Check sheet for the modelled part. Datum: model origin and axes. Units: mm. A direction names the side the tool comes from. Give positions to 0.01 mm unless a question says otherwise; leave off trailing zeros. Write each loop counter-clockwise with the first axis right and the second up, starting at its lowest first coordinate (ties: lowest second). Pieces come first, ordered by that corner, then holes. Notation, with made-up numbers: M 86.5,-11 L 121.5,-11 A25 ccw 121.5,19 Z; hole C 29,76.25 d2. An arc over 180 degrees is marked long. Write item = value, one per line. Start each with the question number.
1) Scan lines: line 1 along Z through (x, y) = (10, 39.5); line 2 along Z through (x, y) = (12, 28); line 3 along Y through (x, z) = (17, 18.75). Record each from-to range of solid material in increasing order. Write a range as [from, to].
2) Mould release check, pull along Y, two halves, no side actions. Record for faces 1 (the flat face through (1, 16.1, 1)), 2 (the flat face through (20, 39, 8)): released by +Y, released by -Y, zero draft, split by the parting line, or undercut.
3) Cross-section at D-D, the plane y = 33. Record the cut outline in (x, z).
4) Cross-section at A-A, the plane x = 10. Record the cut outline in (y, z), plus the area to 3 significant figures.
5) Access from +Z, -Z, +X, -X, +Y, -Y to the whole of each face (thin tool, end or side, straight path). Record for faces 3 (the cylindrical face through (16.88, 16.56, 0.76)), 4 (the cylindrical face through (3.12, 25.24, 0.76)), 5 (the flat face through (0, 39, 8)).
6) Cross-section at C-C, the plane x = 15.5. Record the cut outline in (y, z).
7) Cross-section at B-B, the plane z = 11.5. Record the cut outline in (x, y).
8) Go/stop test with flat-tipped pins: pin 1 (1.5 mm diameter, centred on x = 8, z = 3, fed in from -Y); pin 2 (6 mm diameter, centred on x = 14, y = 14.5, fed in from +Z). Record where each tip stops, or that it passes through.
```python
from build123d import *

# Parameters (mm, degrees)
F1_DEPTH = 1.5
F0_W     = 20
F0_H     = 1.5
F2_DEPTH = 20
F3_R     = 3.75
F4_DEPTH = 25
F5_R     = 1.59999


# Not quite as in the source:
# - a fillet or chamfer is up to 0.001 mm smaller than in the source, because OpenCascade refuses the exact size


with BuildPart() as f1:
    # F0 (on Top) → F1 (new body)
    with BuildSketch(Plane.XY):
        Polygon((0, 3.3), (0, 0), (20, 0), (20, 3.3), (16.4, 3.3), (16.4, 6.5), (20, 6.5), (20, 9.7), (16.4, 9.7), (16.4, 12.9), (20, 12.9), (20, 16.1), (16.4, 16.1), (16.4, 19.3), (20, 19.3), (20, 22.5), (16.4, 22.5), (16.4, 25.7), (20, 25.7), (20, 28.9), (16.4, 28.9), (16.4, 32.1), (20, 32.1), (20, 38.5), (0, 38.5), (0, 32.1), (3.6, 32.1), (3.6, 28.9), (0, 28.9), (0, 25.7), (3.6, 25.7), (3.6, 22.5), (0, 22.5), (0, 19.3), (3.6, 19.3), (3.6, 16.1), (0, 16.1), (0, 12.9), (3.6, 12.9), (3.6, 9.7), (0, 9.7), (0, 6.5), (3.6, 6.5), (3.6, 3.3), align=None)
    extrude(amount=F1_DEPTH)

    # F0 (on Top) → F2 (join)
    with BuildSketch(Plane.XY):
        with Locations((10, 39.25)):
            Rectangle(F0_W, F0_H)
    extrude(amount=F2_DEPTH)

    # F3 (on face) → F4 (cut)
    with BuildSketch(Plane(origin=(0, 40, 0), x_dir=(-1, 0, 0), z_dir=(0, 1, 0))):
        with Locations((-10, 11.5)):
            Circle(F3_R)
    extrude(amount=-F4_DEPTH, mode=Mode.SUBTRACT)

    # F5 (radius 1.6 in the source; OpenCascade refuses exactly that, so slightly less here)
    f5_edges = [f1.edges().sort_by_distance(p)[0] for p in [
        (16.4, 32.1, 0.75),
        (16.4, 28.9, 0.75),
        (16.4, 25.7, 0.75),
        (16.4, 22.5, 0.75),
        (16.4, 16.1, 0.75),
        (16.4, 9.7, 0.75),
        (16.4, 3.3, 0.75),
        (16.4, 19.3, 0.75),
        (16.4, 12.9, 0.75),
        (16.4, 6.5, 0.75),
        (3.6, 32.1, 0.75),
        (3.6, 25.7, 0.75),
        (3.6, 19.3, 0.75),
        (3.6, 12.9, 0.75),
        (3.6, 6.5, 0.75),
        (3.6, 28.9, 0.75),
        (3.6, 22.5, 0.75),
        (3.6, 16.1, 0.75),
        (3.6, 9.7, 0.75),
        (3.6, 3.3, 0.75),
    ]]
    fillet(f5_edges, radius=F5_R)


solid = f1.part
```
Reply:
q1.line_1 = [0, 7.75], [15.25, 20]
q1.line_2 = [0, 1.5]
q1.line_3 = [38.5, 40]
q2.face_1 = undercut
q2.face_2 = zero draft
q3.outline = M 0,0 L 20,0 L 20,1.5 L 0,1.5 Z
q4.outline = M 0,0 L 40,0 L 40,7.75 L 38.5,7.75 L 38.5,1.5 L 0,1.5 Z; M 38.5,15.25 L 40,15.25 L 40,20 L 38.5,20 Z
q4.area = 76.5 mm2
q5.face_3 = +Z, -Z, +X
q5.face_4 = +Z, -Z, -X
q5.face_5 = +Z, -Z, -X, +Y, -Y
q6.outline = M 0,0 L 40,0 L 40,20 L 38.5,20 L 38.5,1.5 L 0,1.5 Z
q7.outline = M 0,38.5 L 6.25,38.5 L 6.25,40 L 0,40 Z; M 13.75,38.5 L 20,38.5 L 20,40 L 13.75,40 Z
q8.pin_1 = 38.5
q8.pin_2 = 1.5
